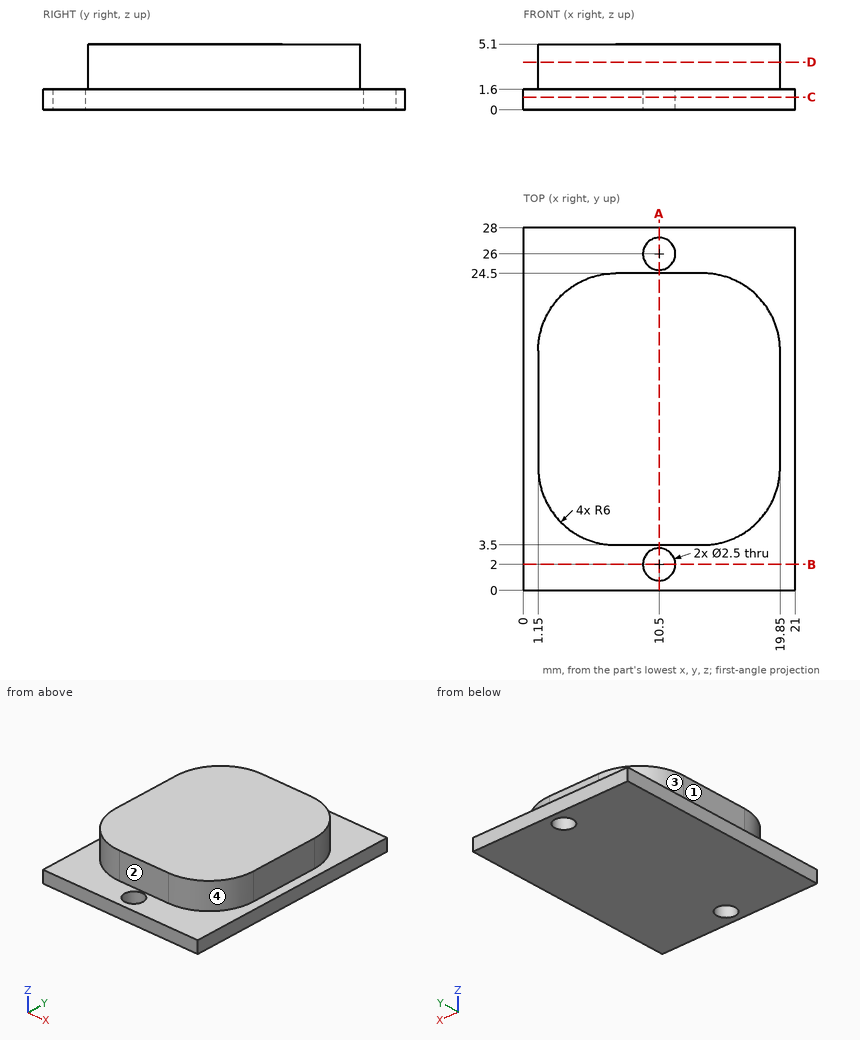
Check sheet for the drawn part. Datum: minimum x, y, z corner. Units: mm. A direction names the side the tool comes from. Give positions to 0.01 mm unless a question says otherwise; leave off trailing zeros. Write each loop counter-clockwise with the first axis right and the second up, starting at its lowest first coordinate (ties: lowest second). Pieces come first, ordered by that corner, then holes. Notation, with made-up numbers: M -17.75,60 L 36.25,60 A22 cw 36.25,91 Z; hole C 2,54 d5. An arc over 180 degrees is marked long. Write item = value, one per line.
(1) Sectioned sample at C-C (z = 1). Record the cut outline in (x, y), then the cut area to 3 significant figures.
Found:
outline = M 0,0 L 21,0 L 21,28 L 0,28 Z; hole C 10.5,2 d2.5; hole C 10.5,26 d2.5
area = 578 mm2
(2) Sectioned sample at A-A (x = 10.5). Record the cut outline in (y, z), then the cut area to 3 significant figures.
Found:
outline = M 0,0 L 0.75,0 L 0.75,1.6 L 0,1.6 Z; M 3.25,0 L 24.75,0 L 24.75,1.6 L 24.5,1.6 L 24.5,5.1 L 3.5,5.1 L 3.5,1.6 L 3.25,1.6 Z; M 27.25,0 L 28,0 L 28,1.6 L 27.25,1.6 Z
area = 110 mm2
(3) Material ranges on line 1 (Y direction, x = 10.5, z = 0.55); line 2 (Z direction, x = 17.25, y = 26); line 3 (Y direction, x = 11.5, z = 3.05), recorded low to high.
Found:
line_1 = 0 to 0.75, 3.25 to 24.75, 27.25 to 28
line_2 = 0 to 1.6
line_3 = 3.5 to 24.5
(4) Access from +Z, -Z, +X, -X, +Y, -Y to the whole of each face (thin tool, end or side, straight path). Record for the marked faces 1, 2, 3 and 4.
Found:
face_1 = +Z, -X, +Y, -Y
face_2 = +Z, +X, -X, -Y
face_3 = +Z, -X, +Y
face_4 = +Z, +X, -Y
(5) Sectioned sample at D-D (z = 3.7). Record the cut outline in (x, y), then the cut area to 3 significant figures.
Found:
outline = M 1.15,9.5 A6 ccw 7.15,3.5 L 13.85,3.5 A6 ccw 19.85,9.5 L 19.85,18.5 A6 ccw 13.85,24.5 L 7.15,24.5 A6 ccw 1.15,18.5 Z
area = 362 mm2
(6) Go/stop test with flat-tipped pins: pin 1 Ø1 at (y, z) = (12.5, 3) entering from -X; pin 2 Ø2 at (x, y) = (10.5, 26) entering from -Z; pin 3 Ø1 at (x, z) = (10, 3) entering from +Y; pin 4 Ø1.7 at (y, z) = (13, 3.5) entering from +X. Record where each tip stops, or that it passes through.
Found:
pin_1 = 1.15
pin_2 = through
pin_3 = 24.5
pin_4 = 19.85
(7) Sectioned sample at B-B (y = 2). Record the cut outline in (x, z), then the cut area to 3 significant figures.
Found:
outline = M 0,0 L 9.25,0 L 9.25,1.6 L 0,1.6 Z; M 11.75,0 L 21,0 L 21,1.6 L 11.75,1.6 Z
area = 29.6 mm2
